Source: CAD feature listing. Evaluate the final solid. Frame: model axes, mm. A direction names the side the tool comes from. Coordinates: 2 decimals unless noted, no trailing zeros. Order: outer loops, then holes, each group sorted by start corner. A loop starts at its lowest first (then second) coordinate and runs counter-clockwise, first axis right, second up.
Item 1: Ray query, line 1 (Y direction, x = 12, z = 23); line 2 (Z direction, x = 8.25, y = 0); line 3 (Z direction, x = 5, y = 114.5). Return the intervals inside material, ascending.
Item 2: Section B-B on y = 98. Return the cut outline in (x, z).
Item 3: Contact query for flat-ended pins moving along their axis: P1, Ø15, axis at x = -3, y = 47, coming from the -Z side; P2, Ø25, axis at x = -10, y = 59.5, coming from the +Z side; P3, Ø19, axis at y = -5.5, z = 24, coming from the +X side. Output: stop coordinate, or through.
Item 4: Mould query, pull axis X, two halves, no side actions, for faces 1 (the flat face through (6, 0, 18)), 2 (the flat face through (-6, 0, 18)), 3 (the flat face through (15, 0, 15)), 4 (the flat face through (-19.844, 52.95, 5.07)). Classes: released by +X, released by -X, zero draft, split by the parting line, or undercut.
Item 5: Section D-D on x = 13. Return the cut outline in (y, z), then the cut area to 3 significant figures.
Item 6: Reachability of faces 5 (the flat face through (10, 12, 17)), 6 (the flat face through (0, 41, 10)), 7 (the cylindrical face through (-5.419, 122.403, 9.65)), 8 (the flat face through (11, 87, 35)) from +Z, -Z, +X, -X, +Y, -Y: full face, straight path, thin tool, end or side. Return the list, or none.
Item 7: Section A-A on y = 0. Return the cut outline in (x, z), then the cut area to 3 significant figures.
Solid Edge part; units mm, degrees
sketch "Sketch1" plane through (0, 0, 0) normal (1, 0, 0) x (0, 1, 0)
  line L0 (-12, 0) -> (-12, 25)
  line L1 (12, 0) -> (12, 25)
  line L2 (0, 0) -> (12, 0)
  line L3 (0, 0) -> (-12, 0)
  arc A0 (-12, 25) -> (12, 25) centre (0, 25) cw
  circle A1 centre (0, 25) radius 6
extrude "Protrusion1" add sketch "Sketch1" along normal blind 15
sketch "Sketch2" plane through (0, 0, 0) normal (1, 0, 0) x (0, 1, 0)
  line L0 (-12, 0) -> (-12, 25)
  line L1 (12, 0) -> (12, 25)
  line L2 (0, 0) -> (12, 0)
  line L3 (0, 0) -> (-12, 0)
  arc A0 (-12, 25) -> (12, 25) centre (0, 25) cw
  circle A1 centre (0, 25) radius 6
extrude "ExtrudedCutout_1" cut sketch "Sketch2" along normal blind 6
sketch "Sketch3" plane through (6, 0, 18.5) normal (-1, 0, 0) x (0, 0, 1)
  line L0 (-8.5, -12) -> (-8.5, 12)
  line L1 (-8.5, 12) -> (-18.5, 12)
  line L2 (-18.5, 12) -> (-18.5, -12)
  line L3 (-18.5, -12) -> (-8.5, -12)
extrude "ExtrudedProtrusion_4" add sketch "Sketch3" along normal blind 6
mirror "Mirror1" about plane through (0, 0, 0) normal (1, 0, 0) of "Protrusion1"
sketch "Sketch4" plane through (6, 0, 18.5) normal (-1, 0, 0) x (0, 0, 1)
  line L0 (-8.5, -12) -> (-8.5, 12)
  line L1 (-8.5, 12) -> (-18.5, 12)
  line L2 (-18.5, 12) -> (-18.5, -12)
  line L3 (-18.5, -12) -> (-8.5, -12)
extrude "ExtrudedCutout_2" cut sketch "Sketch4" along normal blind 12
sketch "Sketch5" plane through (0, 0, 0) normal (1, 0, 0) x (0, 1, 0)
  circle A0 centre (0, 25) radius 6
  line L0 (12, 25) -> (12, 10)
  line L1 (-12, 10) -> (12, 10)
  line L2 (-12, 25) -> (-12, 10)
  arc A1 (-12, 25) -> (12, 25) centre (0, 25) cw
extrude "ExtrudedCutout_3" cut sketch "Sketch5" against normal blind 6
sketch "Sketch6" plane through (6, 0, 18.5) normal (-1, 0, 0) x (0, 0, 1)
  line L0 (-8.5, -12) -> (-8.5, 12)
  line L1 (-8.5, 12) -> (-18.5, 12)
  line L2 (-18.5, 12) -> (-18.5, -12)
  line L3 (-18.5, -12) -> (-8.5, -12)
extrude "ExtrudedProtrusion_6" add sketch "Sketch6" along normal blind 12
sketch "Sketch7" plane through (0, 0, 10) normal (0, 0, 1) x (1, 0, 0)
  line L0 (-15, 12) -> (-24.8246, 95.0638)
  line L1 (0, 98) -> (-24.8246, 95.0638)
  line L2 (0, 98) -> (24.8246, 95.0638)
  line L3 (15, 12) -> (24.8246, 95.0638)
  line L4 (-15, 12) -> (15, 12)
extrude "ExtrudedProtrusion_9" add sketch "Sketch7" against normal blind 10
sketch "Sketch8" plane through (0, 0, 10) normal (0, 0, 1) x (1, 0, 0)
  circle A0 centre (0, 98) radius 24.9976
extrude "Cutout1" cut sketch "Sketch8" against normal blind 17.3955
sketch "Sketch9" plane through (0, 0, 10) normal (0, 0, 1) x (1, 0, 0)
  circle A0 centre (0, 98) radius 24.9976
  circle A1 centre (0, 98) radius 15
extrude "ExtrudedProtrusion_10" add sketch "Sketch9" along normal mid plane 50
Answer list:
1. line 1: y = -12 to -5.66, 5.66 to 12, 76.07 to 89, 107 to 119.93
1. line 2: z = 0 to 19, 31 to 37
1. line 3: z = -15 to 35
2. outline: (-25, -15) - (-15, -15) - (-15, 35) - (-25, 35) - close; (15, -15) - (25, -15) - (25, 35) - (15, 35) - close
3. P1: stops at z = 0
3. P2: stops at z = 10
3. P3: stops at x = 15
4. face 1: undercut
4. face 2: undercut
4. face 3: released by +X
4. face 4: released by -X
5. outline: (-12, 0) - (76.65, 0) - (76.65, -15) - (90.52, -15) - (90.52, 35) - (76.65, 35) - (76.65, 10) - (12, 10) - (12, 25) arc R12 ccw to (-12, 25) - close; (105.48, -15) - (119.35, -15) - (119.35, 35) - (105.48, 35) - close; hole circle Ø12 at (0, 25)
5. area: 2,750 mm2
6. face 5: +Z, +X, -X
6. face 6: +Z
6. face 7: none
6. face 8: +Z, +X, -X, +Y
7. outline: (-15, 0) - (15, 0) - (15, 19) - (6, 19) - (6, 10) - (-6, 10) - (-6, 19) - (-15, 19) - close; (-15, 31) - (-6, 31) - (-6, 37) - (-15, 37) - close; (6, 31) - (15, 31) - (15, 37) - (6, 37) - close
7. area: 570 mm2
